Drawing for the job (mm, zero at the part's lowest x, y, z). A direction names the side the tool comes from. Coordinates: 2 decimals unless noted, no trailing zeros. Loops run counter-clockwise (first coordinate to the right, second up) from the corner with the lowest first, then second, coordinate; pieces in that order, holes last. Notation, with made-up numbers: (86.25, -14) -> (121.25, -14) arc R14 cw to (121.25, 9) -> close; hole circle Ø4 at (66.25, 38.5). An arc over 180 degrees is marked (long way). Write item = value, one per line. Start each with the question number.
(1) Drill centre lines: line 1 (Z direction, x = 305, y = 196); line 2 (X direction, y = 187.5, z = 160.5). Where is each one in solid material? Low to high. Write a range as from..to.
(2) Flat gauge pin, fed straight in: P1, Ø8, axis at x = 457.5, z = 58.5, coming from the -Y side. Where does the tip first touch, or does it go through?
(3) Pull direction Z, two halves, no side cores. Call the marked faces 1, 2 and 3: +Z half, -Z half, draft (parallel to the pull), parting line (faces both ways), or undercut.
(4) Band-saw the part on D-D (z = 335). Write the cut outline in (x, y), and give its area (3 significant figures).
(5) Band-saw the part on C-C (y = 135). Write the cut outline in (x, z).
(6) Band-saw the part on B-B (x = 699). Write the cut outline in (y, z), and give its area (3 significant figures).
(7) Tool access for the marked faces 4 and 5: list every direction of +Z, -Z, +X, -X, +Y, -Y with a clear straight run to the whole face (end or side of a thin tool).
(8) Band-saw the part on A-A (y = 76). Write the cut outline in (x, z).
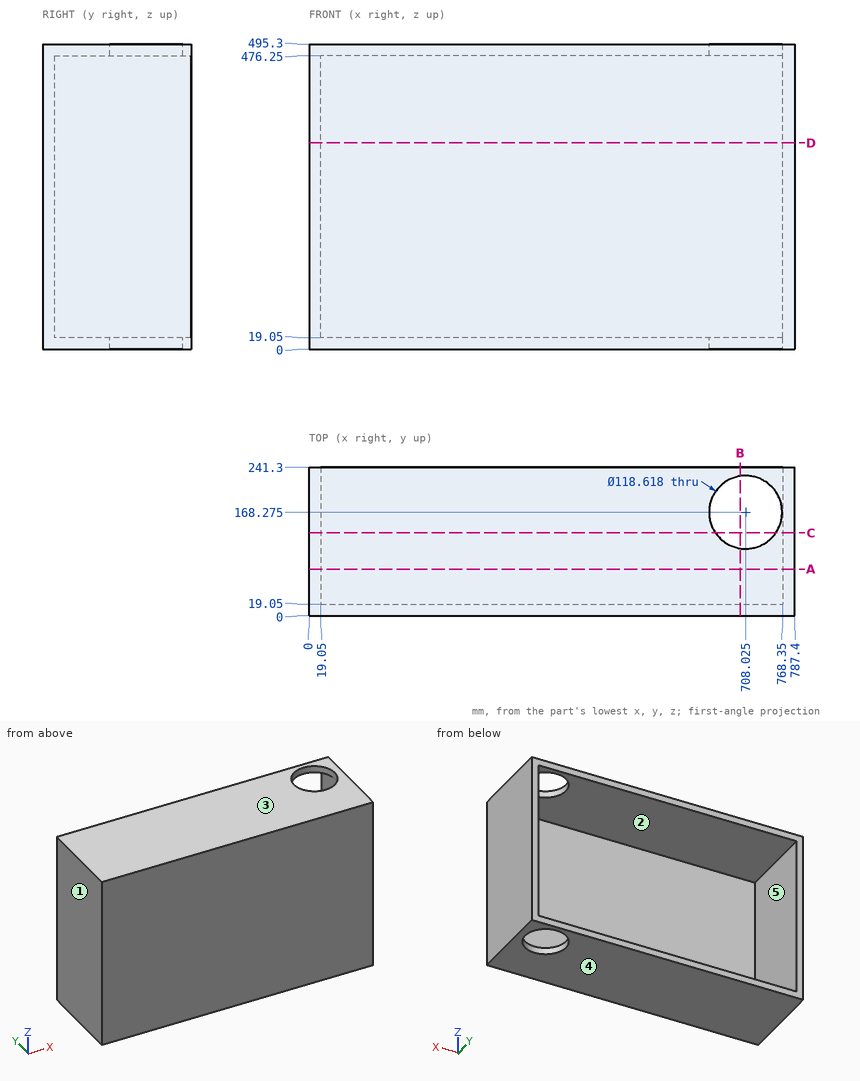
Findings below:
q1.line_1 = 0..19.05, 476.25..495.3
q1.line_2 = 0..19.05, 768.35..787.4
q2.P1 = 0
q3.face_1 = draft
q3.face_2 = undercut
q3.face_3 = +Z half
q4.outline = (0, 0) -> (787.4, 0) -> (787.4, 241.3) -> (768.35, 241.3) -> (768.35, 19.05) -> (19.05, 19.05) -> (19.05, 241.3) -> (0, 241.3) -> close
q4.area = 23,500 mm²
q5.outline = (0, 0) -> (658.93, 0) -> (658.93, 19.05) -> (19.05, 19.05) -> (19.05, 476.25) -> (658.93, 476.25) -> (658.93, 495.3) -> (0, 495.3) -> close; (757.12, 0) -> (787.4, 0) -> (787.4, 495.3) -> (757.12, 495.3) -> (757.12, 476.25) -> (768.35, 476.25) -> (768.35, 19.05) -> (757.12, 19.05) -> close
q6.outline = (0, 0) -> (109.66, 0) -> (109.66, 19.05) -> (19.05, 19.05) -> (19.05, 476.25) -> (109.66, 476.25) -> (109.66, 495.3) -> (0, 495.3) -> close; (226.89, 0) -> (241.3, 0) -> (241.3, 19.05) -> (226.89, 19.05) -> close; (226.89, 476.25) -> (241.3, 476.25) -> (241.3, 495.3) -> (226.89, 495.3) -> close
q6.area = 13,400 mm²
q7.face_4 = -Z, +X, -X, +Y, -Y
q7.face_5 = +Y
q8.outline = (0, 0) -> (787.4, 0) -> (787.4, 495.3) -> (0, 495.3) -> close; hole (19.05, 19.05) -> (768.35, 19.05) -> (768.35, 476.25) -> (19.05, 476.25) -> close
